Design review of the part shown in the three views and the two pictorial views. Dimensions are in mm from the part's minimum x, y and z. Coordinates: 2 decimals unless noted, no trailing zeros. Write each loop counter-clockwise with the first axis right and the second up, starting at its lowest first coordinate (ties: lowest second). Pieces come first, ordered by that corner, then holes.
Q1. For L1, parallel to Z at x = 141.5, y = 3; L2, parallel to Z at x = 25, y = 5.5; L3, parallel to X at y = 3.25, z = 348, list the stretches that pass through material, from the lowest coordinate up.
Q2. Take a section at A-A, the plane x = 448. Write out the cut boundary in (y, z).
Q3. Take a section at B-B, the plane y = 3. Write out the cut boundary in (x, z).
Q4. For pin 1 Ø1 at (y, z) = (3, 423.5) entering from +X; pin 2 Ø3 at (y, z) = (4.5, 256) entering from +X; pin 3 Ø1.9 at (y, z) = (1.5, 376) entering from -X, all flat-tipped, find the tip position at first contact; note any pin that passes through.
Q5. Take a section at C-C, the plane z = 419.5. Write out the cut boundary in (x, y), plus the area to 3 significant figures.
Q6. Take a section at D-D, the plane z = 141. Write out the cut boundary in (x, y).
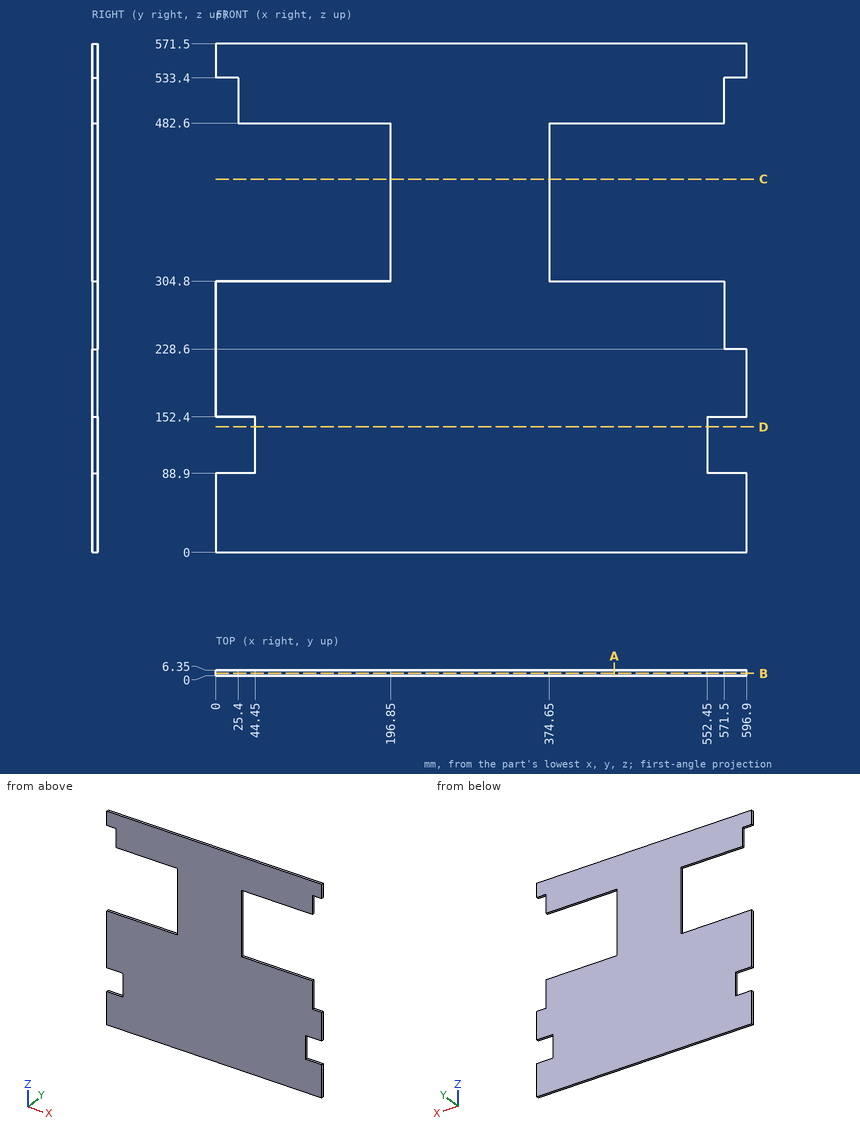
Responses:
1. L1: z = 0 to 304.8, 482.6 to 571.5
1. L2: z = 0 to 88.9, 152.4 to 304.8, 533.4 to 571.5
1. L3: x = 196.85 to 374.65
2. outline: (0, 0) - (6.35, 0) - (6.35, 304.8) - (0, 304.8) - close; (0, 482.6) - (6.35, 482.6) - (6.35, 571.5) - (0, 571.5) - close
3. outline: (0, 0) - (596.9, 0) - (596.9, 88.9) - (552.45, 88.9) - (552.45, 152.4) - (596.9, 152.4) - (596.9, 228.6) - (571.5, 228.6) - (571.5, 304.8) - (374.65, 304.8) - (374.65, 482.6) - (571.5, 482.6) - (571.5, 533.4) - (596.9, 533.4) - (596.9, 571.5) - (0, 571.5) - (0, 533.4) - (25.4, 533.4) - (25.4, 482.6) - (196.85, 482.6) - (196.85, 304.8) - (0, 304.8) - (0, 152.4) - (44.45, 152.4) - (44.45, 88.9) - (0, 88.9) - close
4. pin 1: stops at x = 374.65
4. pin 2: stops at x = 571.5
4. pin 3: stops at x = 196.85
5. outline: (196.85, 0) - (374.65, 0) - (374.65, 6.35) - (196.85, 6.35) - close
5. area: 1,130 mm2
6. outline: (44.45, 0) - (552.45, 0) - (552.45, 6.35) - (44.45, 6.35) - close
